Could you check a few things on this model? Use its own coordinates, in mm. A direction names the side the tool comes from. Round coordinates to 2 decimals unless told otherwise and drop trailing zeros. Loops run counter-clockwise (first coordinate to the right, second up) from the corner with the lowest first, then second, coordinate; pieces in that order, holes last. Notation, with made-up numbers: (-16.75, 26.5) -> (37.25, 26.5) arc R17 ccw to (37.25, 52.5) -> close; hole circle Ø5 at (61.25, 68). An arc over 180 degrees is marked (long way). One line per item, written item: value.
```python
from build123d import *

# Parameters (mm, degrees)
SKETCH1_R           = 40
BOSS_EXTRUDE1_DEPTH = 10
SKETCH2_R           = 24.5
CUT_EXTRUDE1_DEPTH  = 5
BOSS_EXTRUDE2_START = 2
SKETCH3_R           = 30
SKETCH3_R_2         = 24.5
BOSS_EXTRUDE2_DEPTH = 2
SKETCH4_R           = 14
BOSS_EXTRUDE3_DEPTH = 3
SKETCH5_R           = 12.4
BOSS_EXTRUDE4_DEPTH = 12
SKETCH6_R           = 2.05
CUT_EXTRUDE2_DEPTH  = 61
SKETCH7_R           = 5
CUT_EXTRUDE3_DEPTH  = 61
CUT_EXTRUDE6_REACH  = 59.446
SKETCH9_R           = 2.05
CUT_EXTRUDE7_DEPTH  = 3
BOSS_EXTRUDE5_DEPTH = 9


with BuildPart() as part:
    # Sketch1 → Boss-Extrude1 (new body)
    with BuildSketch(Plane(origin=(0, 0, 0), x_dir=(1, 0, 0), z_dir=(0, 1, 0))):
        with Locations(Location((0, 0, 0), (0, 0, 270))):
            Circle(SKETCH1_R)
    extrude(amount=BOSS_EXTRUDE1_DEPTH)

    # Sketch2 → Cut-Extrude1 (cut)
    with BuildSketch(Plane(origin=(0, 10, 0), x_dir=(1, 0, 0), z_dir=(0, 1, 0))):
        with Locations(Location((0, 0, 0), (0, 0, 270))):
            Circle(SKETCH2_R)
    extrude(amount=-CUT_EXTRUDE1_DEPTH, mode=Mode.SUBTRACT)

    # Sketch3 → Boss-Extrude2 (add)
    with BuildSketch(Plane(origin=(0, 10, 0), x_dir=(1, 0, 0), z_dir=(0, 1, 0)).offset(BOSS_EXTRUDE2_START)):
        with Locations(Location((0, 0, 0), (0, 0, 270))):
            Circle(SKETCH3_R)
        with Locations(Location((0, 0, 0), (0, 0, 270))):
            Circle(SKETCH3_R_2, mode=Mode.SUBTRACT)
    extrude(amount=-BOSS_EXTRUDE2_DEPTH)

    # Sketch4 → Boss-Extrude3 (add)
    with BuildSketch(Plane(origin=(0, 5, 0), x_dir=(1, 0, 0), z_dir=(0, 1, 0))):
        with Locations(Location((0, 0, 0), (0, 0, 270))):
            Circle(SKETCH4_R)
    extrude(amount=BOSS_EXTRUDE3_DEPTH)

    # Sketch5 → Boss-Extrude4 (add)
    with BuildSketch(Plane(origin=(0, 8, 0), x_dir=(1, 0, 0), z_dir=(0, 1, 0))):
        with Locations(Location((0, 0, 0), (0, 0, 270))):
            Circle(SKETCH5_R)
    extrude(amount=BOSS_EXTRUDE4_DEPTH)

    # Sketch6 → Cut-Extrude2 (cut, through all)
    with BuildSketch(Plane(origin=(0, 20, 0), x_dir=(1, 0, 0), z_dir=(0, 1, 0))):
        with Locations(Location((-9, 0, 0), (0, 0, 270))):
            Circle(SKETCH6_R)
        with Locations(Location((0, 9, 0), (0, 0, 270))):
            Circle(SKETCH6_R)
        with Locations(Location((9, 0, 0), (0, 0, 270))):
            Circle(SKETCH6_R)
        with Locations(Location((0, -9, 0), (0, 0, 270))):
            Circle(SKETCH6_R)
    extrude(amount=-CUT_EXTRUDE2_DEPTH, mode=Mode.SUBTRACT)

    # Sketch7 → Cut-Extrude3 (cut, through all)
    with BuildSketch(Plane(origin=(0, 20, 0), x_dir=(1, 0, 0), z_dir=(0, 1, 0))):
        with Locations(Location((0, 0, 0), (0, 0, 270))):
            Circle(SKETCH7_R)
    extrude(amount=-CUT_EXTRUDE3_DEPTH, mode=Mode.SUBTRACT)

    # Sketch9 → Cut-Extrude6 (cut, up to next)
    with BuildSketch(Plane(origin=(0, 10, 0), x_dir=(1, 0, 0), z_dir=(0, 1, 0)), mode=Mode.PRIVATE) as cut_extrude6_sk1:
        with Locations(Location((0, 35, 0), (0, 0, 270))):
            Circle(SKETCH9_R)
    cut_extrude6_tool1 = extrude(cut_extrude6_sk1.sketch, amount=-CUT_EXTRUDE6_REACH, mode=Mode.PRIVATE) & part.part
    # Sketch9 → Cut-Extrude6 (cut, up to next)
    with BuildSketch(Plane(origin=(0, 10, 0), x_dir=(1, 0, 0), z_dir=(0, 1, 0)), mode=Mode.PRIVATE) as cut_extrude6_sk2:
        with Locations(Location((35, 0, 0), (0, 0, 270))):
            Circle(SKETCH9_R)
    cut_extrude6_tool2 = extrude(cut_extrude6_sk2.sketch, amount=-CUT_EXTRUDE6_REACH, mode=Mode.PRIVATE) & part.part
    # Sketch9 → Cut-Extrude6 (cut, up to next)
    with BuildSketch(Plane(origin=(0, 10, 0), x_dir=(1, 0, 0), z_dir=(0, 1, 0)), mode=Mode.PRIVATE) as cut_extrude6_sk3:
        with Locations(Location((0, -35, 0), (0, 0, 270))):
            Circle(SKETCH9_R)
    cut_extrude6_tool3 = extrude(cut_extrude6_sk3.sketch, amount=-CUT_EXTRUDE6_REACH, mode=Mode.PRIVATE) & part.part
    # Sketch9 → Cut-Extrude6 (cut, up to next)
    with BuildSketch(Plane(origin=(0, 10, 0), x_dir=(1, 0, 0), z_dir=(0, 1, 0)), mode=Mode.PRIVATE) as cut_extrude6_sk4:
        with Locations(Location((-35, 0, 0), (0, 0, 270))):
            Circle(SKETCH9_R)
    cut_extrude6_tool4 = extrude(cut_extrude6_sk4.sketch, amount=-CUT_EXTRUDE6_REACH, mode=Mode.PRIVATE) & part.part
    # Sketch9 → Cut-Extrude6 (cut, up to next)
    with BuildSketch(Plane(origin=(0, 10, 0), x_dir=(1, 0, 0), z_dir=(0, 1, 0)), mode=Mode.PRIVATE) as cut_extrude6_sk5:
        with Locations(Location((-24.748737342, 24.748737342, 0), (0, 0, 270))):
            Circle(SKETCH9_R)
    cut_extrude6_tool5 = extrude(cut_extrude6_sk5.sketch, amount=-CUT_EXTRUDE6_REACH, mode=Mode.PRIVATE) & part.part
    # Sketch9 → Cut-Extrude6 (cut, up to next)
    with BuildSketch(Plane(origin=(0, 10, 0), x_dir=(1, 0, 0), z_dir=(0, 1, 0)), mode=Mode.PRIVATE) as cut_extrude6_sk6:
        with Locations(Location((24.748737342, 24.748737342, 0), (0, 0, 270))):
            Circle(SKETCH9_R)
    cut_extrude6_tool6 = extrude(cut_extrude6_sk6.sketch, amount=-CUT_EXTRUDE6_REACH, mode=Mode.PRIVATE) & part.part
    # Sketch9 → Cut-Extrude6 (cut, up to next)
    with BuildSketch(Plane(origin=(0, 10, 0), x_dir=(1, 0, 0), z_dir=(0, 1, 0)), mode=Mode.PRIVATE) as cut_extrude6_sk7:
        with Locations(Location((24.748737342, -24.748737342, 0), (0, 0, 270))):
            Circle(SKETCH9_R)
    cut_extrude6_tool7 = extrude(cut_extrude6_sk7.sketch, amount=-CUT_EXTRUDE6_REACH, mode=Mode.PRIVATE) & part.part
    # Sketch9 → Cut-Extrude6 (cut, up to next)
    with BuildSketch(Plane(origin=(0, 10, 0), x_dir=(1, 0, 0), z_dir=(0, 1, 0)), mode=Mode.PRIVATE) as cut_extrude6_sk8:
        with Locations(Location((-24.748737342, -24.748737342, 0), (0, 0, 270))):
            Circle(SKETCH9_R)
    cut_extrude6_tool8 = extrude(cut_extrude6_sk8.sketch, amount=-CUT_EXTRUDE6_REACH, mode=Mode.PRIVATE) & part.part
    add(cut_extrude6_tool1.solids().sort_by_distance((0, 10, -35))[0], mode=Mode.SUBTRACT)
    add(cut_extrude6_tool2.solids().sort_by_distance((35, 10, 0))[0], mode=Mode.SUBTRACT)
    add(cut_extrude6_tool3.solids().sort_by_distance((0, 10, 35))[0], mode=Mode.SUBTRACT)
    add(cut_extrude6_tool4.solids().sort_by_distance((-35, 10, 0))[0], mode=Mode.SUBTRACT)
    add(cut_extrude6_tool5.solids().sort_by_distance((-24.748737, 10, -24.748737))[0], mode=Mode.SUBTRACT)
    add(cut_extrude6_tool6.solids().sort_by_distance((24.748737, 10, -24.748737))[0], mode=Mode.SUBTRACT)
    add(cut_extrude6_tool7.solids().sort_by_distance((24.748737, 10, 24.748737))[0], mode=Mode.SUBTRACT)
    add(cut_extrude6_tool8.solids().sort_by_distance((-24.748737, 10, 24.748737))[0], mode=Mode.SUBTRACT)

    # Sketch10 → Cut-Extrude7 (cut)
    with BuildSketch(Plane(origin=(0, 10, 0), x_dir=(1, 0, 0), z_dir=(0, 1, 0))):
        Polygon((2.044293101, 31.44694511), (4.099182346, 34.993882313), (2.054889246, 38.546937203), (-2.044293101, 38.55305489), (-4.099182346, 35.006117687), (-2.054889246, 31.453062797), align=None)
        Polygon((23.680683804, 20.791137693), (27.642092406, 21.844976021), (28.710145944, 25.802575669), (25.816790879, 28.70633699), (21.855382277, 27.652498662), (20.78732874, 23.694899014), align=None)
        Polygon((31.573449102, -2.24990717), (35.235201316, -4.09243371), (38.661752215, -1.84252654), (38.426550898, 2.24990717), (34.764798684, 4.09243371), (31.338247785, 1.84252654), align=None)
        Polygon((20.739798525, -23.89331762), (22.003452724, -27.792870338), (26.01239154, -28.648290059), (28.757676158, -25.604157063), (27.494021959, -21.704604345), (23.485083143, -20.849184624), align=None)
        Polygon((2.058274344, -31.455026085), (-2.040900294, -31.444995172), (-4.099174638, -34.989969087), (-2.058274344, -38.544973915), (2.040900294, -38.555004828), (4.099174638, -35.010030913), align=None)
        Polygon((-20.760867622, -23.799933658), (-23.576490575, -20.820739015), (-27.564360295, -21.769542699), (-28.736607062, -25.697541025), (-25.920984108, -28.676735668), (-21.933114388, -27.727931984), align=None)
        Polygon((-31.399076536, -1.958745399), (-31.503214993, 2.139118497), (-35.104138457, 4.097863897), (-38.600923464, 1.958745399), (-38.496785007, -2.139118497), (-34.895861543, -4.097863897), align=None)
        Polygon((-23.495263392, 20.845900375), (-20.742044406, 23.882859142), (-21.995518356, 27.785696109), (-26.002211292, 28.651574308), (-28.755430277, 25.614615541), (-27.501956327, 21.711778574), align=None)
    extrude(amount=-CUT_EXTRUDE7_DEPTH, mode=Mode.SUBTRACT)

    # Sketch11 → Boss-Extrude5 (add)
    with BuildSketch(Plane(origin=(0, 10, 0), x_dir=(1, 0, 0), z_dir=(0, 1, 0))):
        with BuildLine():
            Line((9.080620819, -30.218963387), (11.511280004, -38.307837745))
            ThreePointArc((11.511280004, -38.307837745), (15.444999622, -36.897858836), (19.210154537, -35.085181525))
            Line((19.210154537, -35.085181525), (15.153842941, -27.676785701))
            ThreePointArc((15.153842941, -27.676785701), (12.18371763, -29.106707944), (9.080620819, -30.218963387))
        make_face()
    extrude(amount=BOSS_EXTRUDE5_DEPTH)


solid = part.part
```
Item 1: If we mould it in two halves opening along Z, with no side actions, what happens to faces 3 (the face through (0.2, 20, 5.3)), 4 (the face through (-4.88, 10.14, -1.08))? For each: released by +Z, released by -Z, zero draft, split by the parting line, or undercut.
Output:
face 3: zero draft
face 4: undercut
Item 2: Will these pins go through, and if not, where does the flat tip stop? pin 1 Ø3.5 at (x, z) = (-24.75, 24.75) entering from -Y; pin 2 Ø1 at (x, z) = (29, -18) entering from -Y; pin 3 Ø6 at (x, z) = (-35, -2) entering from +Y; pin 4 Ø5 at (x, z) = (13, -24) entering from +Y.
Output:
pin 1: passes through
pin 2: stops at y = 0
pin 3: stops at y = 10
pin 4: stops at y = 12
Item 3: I need wall thicknesses on line 1 (X direction, y = 11.25, z = 0); line 2 (X direction, y = 7, z = -8.5); line 3 (Y direction, x = -25.5, z = -10.5). Which ranges of each line are inside material? Lowest first, please. Write a range as from..to.
Output:
line 1: x = -30..-24.5, -12.4..-11.05, -6.95..-5, 5..6.95, 11.05..12.4, 24.5..30
line 2: x = -39.09..-22.98, -11.12..-1.99, 1.99..11.12, 22.98..39.09
line 3: y = 0..12
Item 4: If we section it at B-B on x = 0: Count the separate pieces of the cut face and the enclosed holes in it, plus the area to 3 significant figures.
Output:
separate pieces: 6
enclosed holes: 0
area: 495 mm²
Item 5: For faces 1 (the face through (21.33, 8.52, -25.7)), 2 (the face through (-24.7, 3.5, 22.7)), which set-ups out of +Z, -Z, +X, -X, +Y, -Y let a thin tool reach every point of the face, with its end or its side?
Output:
face 1: +Y
face 2: +Y, -Y
Item 6: If we section it at A-A on z = 9: List the corners of the cut face in (x, y) for me.
Output:
outline: (-38.97, 0) -> (-2.05, 0) -> (-2.05, 20) -> (-8.53, 20) -> (-8.53, 8) -> (-10.72, 8) -> (-10.72, 5) -> (-22.79, 5) -> (-22.79, 12) -> (-28.62, 12) -> (-28.62, 10) -> (-38.97, 10) -> close; (2.05, 0) -> (38.97, 0) -> (38.97, 10) -> (28.62, 10) -> (28.62, 12) -> (22.79, 12) -> (22.79, 5) -> (10.72, 5) -> (10.72, 8) -> (8.53, 8) -> (8.53, 20) -> (2.05, 20) -> close
